from build123d import *

# Parameters (mm, degrees)
IZIM1_R                                           = 29
Y_KSEKLIK_EKSTR_ZYON1_DEPTH                       = 64.5
IZIM2_R                                           = 17.5
KES_EKSTR_ZYON1_DEPTH                             = 59.5
F_5_0_5_AP_DELIK1_D                               = 5
F_5_0_5_AP_DELIK1_DEPTH                           = 6
F_5_0_5_AP_DELIK1_TIP                             = 0.909925586
PAH1_SIZE                                         = 0.5
PAH2_SIZE                                         = 1
KES_EKSTR_ZYON2_DEPTH                             = 92.461740635
IZIM15_W                                          = 3
IZIM15_H                                          = 10
KES_EKSTR_ZYON4_DEPTH                             = 92.461740801
M5_ALT_GEN_ALYAN_BA_L_K_R_VIDA_IN_HAV_D           = 5.2
M5_ALT_GEN_ALYAN_BA_L_K_R_VIDA_IN_HAV_DEPTH       = 87.053677391
M5_ALT_GEN_ALYAN_BA_L_K_R_VIDA_IN_HAV_CBORE_D     = 9
M5_ALT_GEN_ALYAN_BA_L_K_R_VIDA_IN_HAV_CBORE_DEPTH = 6
M5_ALT_GEN_ALYAN_BA_L_K_R_VIDA_IN_HAV_TIP         = 0.946322609


with BuildPart() as part:
    # Çizim1 → Yükseklik-Ekstrüzyon1 (new body)
    with BuildSketch(Plane(origin=(0, 0, 0), x_dir=(1, 0, 0), z_dir=(0, 1, 0))):
        with Locations(Location((0, 0, 0), (0, 0, 270))):
            Circle(IZIM1_R)
    extrude(amount=Y_KSEKLIK_EKSTR_ZYON1_DEPTH)

    # Çizim2 → Kes-Ekstrüzyon1 (cut)
    with BuildSketch(Plane(origin=(0, 64.5, 0), x_dir=(1, 0, 0), z_dir=(0, 1, 0))):
        with Locations(Location((0, 0, 0), (0, 0, 270))):
            Circle(IZIM2_R)
    extrude(amount=-KES_EKSTR_ZYON1_DEPTH, mode=Mode.SUBTRACT)

    # Ø5.0 (5) Çap Delik1
    with Locations(Plane(origin=(0, 0, 0), x_dir=(-1, 0, 0), z_dir=(0, -1, 0))):
        with Locations((0, 0)):
            Hole(F_5_0_5_AP_DELIK1_D / 2, depth=F_5_0_5_AP_DELIK1_DEPTH)
            with Locations((0, 0, -(F_5_0_5_AP_DELIK1_DEPTH + F_5_0_5_AP_DELIK1_TIP / 2))):  # 140° drill point
                Cone(0, F_5_0_5_AP_DELIK1_D / 2, F_5_0_5_AP_DELIK1_TIP, mode=Mode.SUBTRACT)

    # Pah1
    pah1_edges = [part.edges().sort_by_distance(p)[0] for p in [
        (-2.5, 0, 0),
    ]]
    chamfer(pah1_edges, length=PAH1_SIZE)

    # Pah2
    pah2_edges = [part.edges().sort_by_distance(p)[0] for p in [
        (-2.5, 5, 0),
    ]]
    chamfer(pah2_edges, length=PAH2_SIZE)

    # Çizim6 → Kes-Ekstrüzyon2 (cut, through all)
    with BuildSketch(Plane.XY.offset(29)):
        with BuildLine():
            Line((-1.5, 53.5), (-1.5, 55.5))
            ThreePointArc((-1.5, 55.5), (0, 57), (1.5, 55.5))
            Line((1.5, 55.5), (1.5, 53.5))
            ThreePointArc((1.5, 53.5), (0, 52), (-1.5, 53.5))
        make_face()
    extrude(amount=-KES_EKSTR_ZYON2_DEPTH, mode=Mode.SUBTRACT)

    # Çizim15 → Kes-Ekstrüzyon4 (cut, through all)
    with BuildSketch(Plane.XY.offset(29)):
        with Locations((0, 59.5)):
            Rectangle(IZIM15_W, IZIM15_H)
    extrude(amount=-KES_EKSTR_ZYON4_DEPTH, mode=Mode.SUBTRACT)

    # M5 Altıgen Alyan Başlı Kör Vida İçin Havşa2
    with Locations(Plane(origin=(11.75, 0, 20.351596989), x_dir=(0, 0, -1), z_dir=(0, -1, 0))):
        with Locations((0, 0), (40.703193978, 0), (20.351596989, -35.25)):
            CounterBoreHole(M5_ALT_GEN_ALYAN_BA_L_K_R_VIDA_IN_HAV_D / 2, M5_ALT_GEN_ALYAN_BA_L_K_R_VIDA_IN_HAV_CBORE_D / 2, M5_ALT_GEN_ALYAN_BA_L_K_R_VIDA_IN_HAV_CBORE_DEPTH, depth=M5_ALT_GEN_ALYAN_BA_L_K_R_VIDA_IN_HAV_DEPTH)
            with Locations((0, 0, -(M5_ALT_GEN_ALYAN_BA_L_K_R_VIDA_IN_HAV_DEPTH + M5_ALT_GEN_ALYAN_BA_L_K_R_VIDA_IN_HAV_TIP / 2))):  # 140° drill point
                Cone(0, M5_ALT_GEN_ALYAN_BA_L_K_R_VIDA_IN_HAV_D / 2, M5_ALT_GEN_ALYAN_BA_L_K_R_VIDA_IN_HAV_TIP, mode=Mode.SUBTRACT)


solid = part.part
Model file for the job. Use its own axes, mm. A direction names the side the tool comes from. Give positions to 0.01 mm unless a question says otherwise; leave off trailing zeros. Write each loop counter-clockwise with the first axis right and the second up, starting at its lowest first coordinate (ties: lowest second). Pieces come first, ordered by that corner, then holes. Notation, with made-up numbers: M 3.25,33.5 L 35.25,33.5 A17 ccw 35.25,44.5 Z; hole C 47.25,50 d5. An arc over 180 degrees is marked long. One line per item, written item: value. Start each with the question number.
Q1. Probe probe 1 along X at (y, z) = (44, 0); probe 2 along X at (y, z) = (17.5, -2); probe 3 along Z at (x, y) = (14, 44). List the from-to ranges inside material, lowest first. Write a range as [from, to].
Q2. Saw through at C-C, the plane y = 10. Write the cut outline in (x, z).
Q3. Drop flat-ended pins along their axis: pin 1 Ø5 at (y, z) = (20, 13) entering from -X; pin 2 Ø12 at (y, z) = (60, 21.5) entering from +X; pin 3 Ø4 at (x, z) = (0, 0) entering from -Y; pin 4 Ø7 at (x, z) = (11.75, 20.35) entering from -Y. Give the stop position or say it passes through.
Q4. Saw through at D-D, the plane x = 11.75. Write the cut outline in (y, z), plus the area to 3 significant figures.
Q5. Saw through at A-A, the plane z = 0. Write the cut outline in (x, y).
Q6. Two-plate mould, pull along Z, no slides. Class faces 1 (the flat face through (1.5, 59, 23)), 2 (the cylindrical face through (-11.107, 31.798, 26.789)), 3 (the flat face through (-4, 5, 0)): +Z half, -Z half, draft (parallel to the pull), parting line (faces both ways), or undercut.
Q7. 3-axis set-ups, long thin cutter, end or side, ignore diameter. For faces 4 (the flat face through (-1.5, 59, 23)), 5 (the flat face through (-18, 64.5, 0)), 6 (the cylindrical face through (9.443, 35.66, 21.551)), 7 (the flat face through (10, 6, 18)), 8 (the cylindrical face through (5.26, 35.17, 16.69)): which of +Z, -Z, +X, -X, +Y, -Y reach the whole face in a straight line?
Q8. Saw through at B-B, the plane x = 0. Write the cut outline in (y, z).
Output values:
1. probe 1: x = [-29, -26.1], [-20.9, -17.5], [17.5, 29]
1. probe 2: x = [-28.93, -25.16], [-21.84, -17.39], [17.39, 28.93]
1. probe 3: z = [-25.4, -21.65], [-19.05, -10.5], [10.5, 19.05], [21.65, 25.4]
2. outline: C 0,0 d58; hole C -23.5,0 d5.2; hole C 0,0 d35; hole C 11.75,-20.35 d5.2; hole C 11.75,20.35 d5.2
3. pin 1: stops at x = -27.03
3. pin 2: stops at x = 24.51
3. pin 3: passes through
3. pin 4: stops at y = 6
4. outline: M 0,-26.51 L 64.5,-26.51 L 64.5,-22.95 L 6,-22.95 L 6,-24.85 L 0,-24.85 Z; M 0,-15.85 L 6,-15.85 L 6,-17.75 L 64.5,-17.75 L 64.5,-12.97 L 5,-12.97 L 5,12.97 L 64.5,12.97 L 64.5,17.75 L 6,17.75 L 6,15.85 L 0,15.85 Z; M 0,24.85 L 6,24.85 L 6,22.95 L 64.5,22.95 L 64.5,26.51 L 0,26.51 Z
4. area: 1,160 mm²
5. outline: M -29,0 L -28,0 L -28,6 L -26.1,6 L -26.1,64.5 L -29,64.5 Z; M -20.9,6 L -19,6 L -19,0 L -3,0 L -2.5,0.5 L -2.5,4 L -3.5,5 L -17.5,5 L -17.5,64.5 L -20.9,64.5 Z; M 2.5,0.5 L 3,0 L 29,0 L 29,64.5 L 17.5,64.5 L 17.5,5 L 3.5,5 L 2.5,4 Z
6. face 1: draft
6. face 2: parting line
6. face 3: undercut
7. face 4: +Z, -Z, +Y
7. face 5: +Z, -Z, +X, -X, +Y
7. face 6: +Y, -Y
7. face 7: -Y
7. face 8: +Y
8. outline: M 0,-29 L 52,-29 L 52,-17.5 L 5,-17.5 L 5,-3.5 L 4,-2.5 L 0.5,-2.5 L 0,-3 Z; M 0,3 L 0.5,2.5 L 4,2.5 L 5,3.5 L 5,17.5 L 52,17.5 L 52,29 L 0,29 Z
